Design review of the part built by this model. Coordinates are the model's own, in mm. A direction names the side the tool comes from. Round coordinates to 2 decimals unless told otherwise and drop trailing zeros. Loops run counter-clockwise (first coordinate to the right, second up) from the corner with the lowest first, then second, coordinate; pieces in that order, holes last. Notation, with made-up numbers: (-18.75, 63.5) - (-12.75, 63.5) arc R13 cw to (-12.75, 85.5) - close; hole circle Ø7 at (31.5, -12). An arc over 180 degrees is marked (long way). Return JSON: item names as keys, results as strings. Group by question number.
from build123d import *

# Parameters (mm, degrees)
SKETCH1_W                      = 32
SKETCH1_H                      = 20
SKETCH1_R                      = 1.5
BOSS_EXTRUDE1_DEPTH            = 10
CBORE_FOR_M5_SHCS1_D           = 5.3
CBORE_FOR_M5_SHCS1_CBORE_D     = 9.5
CBORE_FOR_M5_SHCS1_CBORE_DEPTH = 5
SKETCH7_W                      = 3
SKETCH7_H                      = 20
CUT_EXTRUDE1_DEPTH             = 3
CHAMFER1_SIZE                  = 0.5
CHAMFER2_SIZE                  = 0.1


with BuildPart() as part:
    # Sketch1 → Boss-Extrude1 (new body)
    with BuildSketch(Plane(origin=(0, 0, 0), x_dir=(1, 0, 0), z_dir=(0, 1, 0))):
        with Locations((1.866408356, 4.25)):
            Rectangle(SKETCH1_W, SKETCH1_H)
        with Locations(Location((-4.133591644, 4.25, 0), (0, 0, 270))):
            Circle(SKETCH1_R, mode=Mode.SUBTRACT)
        with Locations(Location((9.866408356, 4.25, 0), (0, 0, 270))):
            Circle(SKETCH1_R, mode=Mode.SUBTRACT)
    extrude(amount=BOSS_EXTRUDE1_DEPTH)

    # CBORE for M5 SHCS1 (through all)
    with Locations(Plane(origin=(0, 10, 0), x_dir=(1, 0, 0), z_dir=(0, 1, 0))):
        with Locations((-4.133591644, 4.25), (9.866408356, 4.25)):
            CounterBoreHole(CBORE_FOR_M5_SHCS1_D / 2, CBORE_FOR_M5_SHCS1_CBORE_D / 2, CBORE_FOR_M5_SHCS1_CBORE_DEPTH)

    # Sketch7 → Cut-Extrude1 (cut)
    with BuildSketch(Plane(origin=(0, 10, 0), x_dir=(1, 0, 0), z_dir=(0, 1, 0))):
        with Locations((-12.633591644, 4.25)):
            Rectangle(SKETCH7_W, SKETCH7_H)
    extrude(amount=-CUT_EXTRUDE1_DEPTH, mode=Mode.SUBTRACT)

    # Chamfer1
    chamfer1_edges = [part.edges().sort_by_distance(p)[0] for p in [
        (17.866408356, 10, -4.25),
        (3.366408356, 10, -14.25),
        (5.116408356, 10, -4.25),
        (-8.883591644, 10, -4.25),
        (3.366408356, 10, 5.75),
        (-11.133591644, 10, -4.25),
    ]]
    chamfer(chamfer1_edges, length=CHAMFER1_SIZE)

    # Chamfer2
    chamfer2_edges = [part.edges().sort_by_distance(p)[0] for p in [
        (12.516408356, 0, -4.25),
        (-1.483591644, 0, -4.25),
        (-14.133591644, 3.5, -14.25),
        (-14.133591644, 3.5, 5.75),
        (-14.133591644, 7, -4.25),
        (-12.633591644, 7, -14.25),
        (-11.133591644, 8.25, -14.25),
        (-12.633591644, 7, 5.75),
        (-11.133591644, 8.25, 5.75),
        (1.866408356, 0, -14.25),
        (17.866408356, 0, -4.25),
        (1.866408356, 0, 5.75),
        (-14.133591644, 0, -4.25),
        (17.866408356, 4.75, 5.75),
        (17.866408356, 4.75, -14.25),
    ]]
    chamfer(chamfer2_edges, length=CHAMFER2_SIZE)


solid = part.part
Q1. Add section A-A, the plane y = 6.25. State the section outline as (x, z) points, plus the area to 3 significant figures.
Q2. Tool access review of faces 4 (the flat face through (-13, 7, -4)), 5 (the flat face through (3, 10, -4)), 6 (the cylindrical face through (6.4, 7.3, -7.5)): name each direction out of +Z, -Z, +X, -X, +Y, -Y from which nothing blocks a thin tool from reaching the whole face with its end or side.
Q3. Add section B-B, the plane z = 2. State the section outline as (x, y) points, plus the area to 3 significant figures.
Q4. Draft analysis for pull direction Z (two halves, no side actions). For faces 1 (the flat face through (2, 5, -14.25)), 2 (the flat face through (2, 5, 5.75)), 3 (the flat face through (-2, 5, -2)), state which applies: pulls with the +Z half, pulls with the -Z half, needs draft (parallel to the pull), parting line crosses it, or undercut.
Q5. Insertion check: pin 1 Ø10.5 at (x, z) = (-5, -4) entering from +Y; pin 2 Ø1.5 at (x, z) = (6, -4.5) entering from +Y; pin 3 Ø3 at (x, z) = (-13, -2.5) entering from +Y. Each pin has a flat end and moves straight along its axis. Give the tip position at first contact, or say it passes through.
Q6. For line 1 (X direction, y = 8.5, z = -4.25); line 2 (X direction, y = 6.7, z = -4.25); line 3 (Y direction, x = -8.5, z = -5.5), list the stretches that pass through material, from the lowest coordinate up.
Q7. Add section C-C, the plane z = -4.25. Give the number of separate pieces and of enclosed holes in the cut face, plus the area to 3 significant figures.
Evaluation:
{
 "1": {"outline": "(-14.13, -14.15) - (-14.03, -14.25) - (17.77, -14.25) - (17.87, -14.15) - (17.87, 5.65) - (17.77, 5.75) - (-14.03, 5.75) - (-14.13, 5.65) - close; hole circle Ø9.5 at (-4.13, -4.25); hole circle Ø9.5 at (9.87, -4.25)", "area": "498 mm²"},
 "2": {"face 4": "+Z, -Z, -X, +Y", "face 5": "+Z, -Z, +X, -X, +Y", "face 6": "+Y"},
 "3": {"outline": "(-14.13, 0.1) - (-14.03, 0) - (17.77, 0) - (17.87, 0.1) - (17.87, 9.5) - (17.37, 10) - (-10.63, 10) - (-11.13, 9.5) - (-11.13, 7) - (-14.03, 7) - (-14.13, 6.9) - close", "area": "311 mm²"},
 "4": {"face 1": "pulls with the -Z half", "face 2": "pulls with the +Z half", "face 3": "undercut"},
 "5": {"pin 1": "y = 10", "pin 2": "y = 5", "pin 3": "y = 7"},
 "6": {"line 1": "-11.13 to -8.88, 0.62 to 5.12, 14.62 to 17.87", "line 2": "-14.13 to -8.88, 0.62 to 5.12, 14.62 to 17.87", "line 3": "0 to 5"},
 "7": {"separate pieces": "3", "enclosed holes": "0", "area": "162 mm²"}
}
